```python
from build123d import *

# Parameters (mm, degrees)
SKETCH1_W           = 200
SKETCH1_H           = 200
BOSS_EXTRUDE1_DEPTH = 5
SKETCH2_R           = 2.125
CUT_EXTRUDE1_DEPTH  = 283.886903196
FILLET1_R           = 5
CHAMFER1_SIZE       = 1
CHAMFER2_SIZE       = 0.5


with BuildPart() as part:
    # Sketch1 → Boss-Extrude1 (new body)
    with BuildSketch(Plane(origin=(0, 0, 0), x_dir=(1, 0, 0), z_dir=(0, 1, 0))):
        with Locations((-100, -100)):
            Rectangle(SKETCH1_W, SKETCH1_H)
    extrude(amount=BOSS_EXTRUDE1_DEPTH)

    # Sketch2 → Cut-Extrude1 (cut, through all)
    with BuildSketch(Plane(origin=(0, 5, 0), x_dir=(1, 0, 0), z_dir=(0, 1, 0))):
        with Locations(Location((-185.303300859, -185.303300859, 0), (0, 0, 270))):
            Circle(SKETCH2_R)
        with Locations(Location((-174.696699141, -174.696699141, 0), (0, 0, 270))):
            Circle(SKETCH2_R)
        with Locations(Location((-185.303300859, -14.692576694, 0), (0, 0, 270))):
            Circle(SKETCH2_R)
        with Locations(Location((-174.696699141, -25.299178412, 0), (0, 0, 270))):
            Circle(SKETCH2_R)
        with Locations(Location((-14.692576694, -14.692576694, 0), (0, 0, 270))):
            Circle(SKETCH2_R)
        with Locations(Location((-25.299178412, -25.299178412, 0), (0, 0, 270))):
            Circle(SKETCH2_R)
        with Locations(Location((-14.692576694, -185.303300859, 0), (0, 0, 270))):
            Circle(SKETCH2_R)
        with Locations(Location((-25.299178412, -174.696699141, 0), (0, 0, 270))):
            Circle(SKETCH2_R)
    extrude(amount=-CUT_EXTRUDE1_DEPTH, mode=Mode.SUBTRACT)

    # Fillet1
    fillet1_edges = [part.edges().sort_by_distance(p)[0] for p in [
        (0, 2.5, 200),
        (-200, 2.5, 200),
        (-200, 2.5, 0),
        (0, 2.5, 0),
    ]]
    fillet(fillet1_edges, radius=FILLET1_R)

    # Chamfer1
    chamfer1_edges = [part.edges().sort_by_distance(p)[0] for p in [
        (-200, 5, 100),
        (-100, 5, 0),
        (0, 5, 100),
        (-100, 5, 200),
        (-198.535533906, 5, 198.535533906),
        (-1.464466094, 5, 198.535533906),
        (-1.464466094, 5, 1.464466094),
        (-198.535533906, 5, 1.464466094),
    ]]
    chamfer(chamfer1_edges, length=CHAMFER1_SIZE)

    # Chamfer2
    chamfer2_edges = [part.edges().sort_by_distance(p)[0] for p in [
        (-200, 0, 100),
        (0, 0, 100),
        (-100, 0, 200),
        (-100, 0, 0),
        (-198.535533906, 0, 198.535533906),
        (-1.464466094, 0, 198.535533906),
        (-1.464466094, 0, 1.464466094),
        (-198.535533906, 0, 1.464466094),
    ]]
    chamfer(chamfer2_edges, length=CHAMFER2_SIZE)


solid = part.part
```
The model under review builds one solid part; all positions refer to its coordinate system, in mm. Coordinates: 2 decimals unless noted, no trailing zeros. One line per item, written item: value. Start each with the question number.
Q1. The part is to be moulded in two halves that separate along Z. For faces 1 (the face through (-2, 2, 1)), 2 (the face through (-183.511, 2.535, 186.446)), 3 (the face through (-197.99, 4.73, 198.05)), say which applies: +Z half, -Z half, draft (parallel to the pull), parting line (faces both ways), or undercut.
Q2. To check wall thickness, follow probe 1 along X at (y, z) = (1.7, 175); probe 2 along Z at (x, y) = (-16.5, 0.85); probe 3 along X at (y, z) = (4.1, 148). State the ranges of each line that lie inside material, in increasing order.
Q3. Clearance check with flat-ended pins moving along their axes: P1, Ø3.5, axis at x = -174.7, z = 25.3, coming from the +Y side; P2, Ø7, axis at x = -174.7, z = 174.7, coming from the +Y side. State where each tip first meets the part, or that it passes through.
Response:
1. face 1: -Z half
1. face 2: undercut
1. face 3: +Z half
2. probe 1: -200 to -176.8, -172.59 to -27.4, -23.2 to 0
2. probe 2: 0 to 13.58, 15.81 to 184.19, 186.42 to 200
2. probe 3: -199.9 to -0.1
3. P1: through
3. P2: y = 5
